from build123d import *

# Parameters (mm, degrees)
F1_DEPTH = 6
F2_R     = 1.55
F3_DEPTH = 6
F4_R     = 1.65
F5_DEPTH = 6


with BuildPart() as f1:
    # F0 (on Front) → F1 (new body)
    with BuildSketch(Plane.XZ):
        with BuildLine():
            Line((0, 6), (0, 0))
            Line((0, 0), (6, 0))
            ThreePointArc((6, 0), (6.433861, 0.047626), (6.847059, 0.188235))
            Line((6.847059, 0.188235), (14.597386, 3.811765))
            ThreePointArc((14.597386, 3.811765), (15.010584, 3.952374), (15.444444, 4))
            Line((15.444444, 4), (19, 4))
            ThreePointArc((19, 4), (20.414214, 4.585786), (21, 6))
            Line((21, 6), (21, 8))
            ThreePointArc((21, 8), (20.414214, 9.414214), (19, 10))
            Line((19, 10), (15.444444, 10))
            ThreePointArc((15.444444, 10), (15.010584, 9.952374), (14.597386, 9.811765))
            Line((14.597386, 9.811765), (6.847059, 6.188235))
            ThreePointArc((6.847059, 6.188235), (6.433861, 6.047626), (6, 6))
            Line((6, 6), (0, 6))
        make_face()
    extrude(amount=F1_DEPTH)

    # F2 (on face) → F3 (cut, through all)
    with BuildSketch(Plane.XY.offset(6)):
        with Locations((3, -3)):
            Circle(F2_R)
    extrude(amount=-F3_DEPTH, mode=Mode.SUBTRACT)

    # F4 (on face) → F5 (cut, through all)
    with BuildSketch(Plane.XZ.offset(6)):
        with Locations((17.222222, 7)):
            Circle(F4_R)
    extrude(amount=-F5_DEPTH, mode=Mode.SUBTRACT)


solid = f1.part
Geometry: final body of the model. Coordinates: model frame, mm. A direction names the side the tool comes from. Round coordinates to 2 decimals unless told otherwise and drop trailing zeros. Order: outer loops, then holes, each group sorted by start corner. A loop starts at its lowest first (then second) coordinate and runs counter-clockwise, first axis right, second up. Notation, with made-up numbers: (14, -37.75) - (53, -37.75) arc R18 ccw to (53, -32.75) - close; hole circle Ø8 at (14.25, 62). An arc over 180 degrees is marked (long way). Write each question's results on one line, items separated by ' | '.
Item 1: Section A-A, the plane y = -3. Return the cut outline in (x, z).
Completed:
outline: (0, 0) - (1.45, 0) - (1.45, 6) - (0, 6) - close; (4.55, 0) - (6, 0) arc R2 ccw to (6.85, 0.19) - (14.6, 3.81) arc R2 cw to (15.44, 4) - (19, 4) arc R2 ccw to (21, 6) - (21, 8) arc R2 ccw to (19, 10) - (15.44, 10) arc R2 ccw to (14.6, 9.81) - (6.85, 6.19) arc R2 cw to (6, 6) - (4.55, 6) - close; hole circle Ø3.3 at (17.22, 7)
Item 2: First-contact query: pin 1 Ø3 at (x, y) = (3, -3) entering from -Z; pin 2 Ø3 at (x, y) = (17, -4) entering from -Z. Flat tips, straight axial feed; report the tip coordinate or a pass-through.
Completed:
pin 1: through | pin 2: z = 4
Item 3: Material intervals for line 1 along Y through (x, z) = (3, 3.45); line 2 along Z through (x, y) = (17.25, -0.45); line 3 along Z through (x, y) = (16, -4.35), sorted ascending. Write a range as [from, to].
Completed:
line 1: [-6, -4.55], [-1.45, 0] | line 2: [4, 5.35], [8.65, 10] | line 3: [4, 5.89], [8.11, 10]
Item 4: Mould query, pull axis X, two halves, no side actions, for faces 4 (the flat face through (10, 0, 5)), 5 (the cylindrical face through (20.43, -2.96, 9.4)), 6 (the cylindrical face through (1.45, -2.93, 3.04)). Classes: pulls with the +X half, pulls with the -X half, needs draft (parallel to the pull), parting line crosses it, or undercut.
Completed:
face 4: needs draft | face 5: pulls with the +X half | face 6: undercut
Item 5: Section C-C, the plane z = 7. Return the cut outline in (x, y), and give its area (3 significant figures).
Completed:
outline: (8.58, -6) - (15.57, -6) - (15.57, 0) - (8.58, 0) - close; (18.87, -6) - (21, -6) - (21, 0) - (18.87, 0) - close | area: 54.7 mm^2
Item 6: Section D-D, the plane y = -4.85. Return the cut outline in (x, z).
Completed:
outline: (0, 0) - (6, 0) arc R2 ccw to (6.85, 0.19) - (14.6, 3.81) arc R2 cw to (15.44, 4) - (19, 4) arc R2 ccw to (21, 6) - (21, 8) arc R2 ccw to (19, 10) - (15.44, 10) arc R2 ccw to (14.6, 9.81) - (6.85, 6.19) arc R2 cw to (6, 6) - (0, 6) - close; hole circle Ø3.3 at (17.22, 7)
Item 7: Reachability of faces 1 (the flat face through (17, -3, 4)), 2 (the flat face through (4.4, -1.6, 6)), 3 (the flat face through (1.6, -1.6, 0)) from +Z, -Z, +X, -X, +Y, -Y: full face, straight path, thin tool, end or side. Return the list, or none.
Completed:
face 1: -Z, +X, +Y, -Y | face 2: +Z, -X, +Y, -Y | face 3: -Z, +X, -X, +Y, -Y
Item 8: Section B-B, the plane x = 3. Return the cut outline in (y, z).
Completed:
outline: (-6, 0) - (-4.55, 0) - (-4.55, 6) - (-6, 6) - close; (-1.45, 0) - (0, 0) - (0, 6) - (-1.45, 6) - close
